Geometry: see drawing. Coordinates: mm, zero at the bounding-box minimum. Round coordinates to 2 decimals unless told otherwise and drop trailing zeros. Loops run counter-clockwise (first coordinate to the right, second up) from the corner with the lowest first, then second, coordinate; pieces in that order, holes last. Notation, with made-up numbers: (61.5, 43) - (77.5, 43) arc R15 cw to (77.5, 67) - close; hole circle Ø5 at (-19, -35). An arc over 180 degrees is marked (long way). Return JSON: item names as keys, results as strings. Group by question number.
1. Section B-B on y = 1. Return loops of the section in (x, z), and give its area (3 significant figures).
2. Section A-A on y = 6.25. Return loops of the section in (x, z).
3. First-contact query: pin 1 Ø1 at (y, z) = (3, 12.5) entering from -X; pin 2 Ø1 at (y, z) = (2.5, 3.5) entering from -X. Flat tips, straight axial feed; report the tip coordinate or a pass-through.
4. Draft query along Z for the marked faces 1, 2, 3 and 4. Return one class per face: +Z half, -Z half, draft (parallel to the pull), parting line (faces both ways), or undercut.
5. Material intervals for probe 1 along Z at (x, y) = (7.5, 4.6); probe 2 along Y at (x, z) = (8.5, 7); probe 3 along X at (y, z) = (5.5, 9.5), sorted ascending.
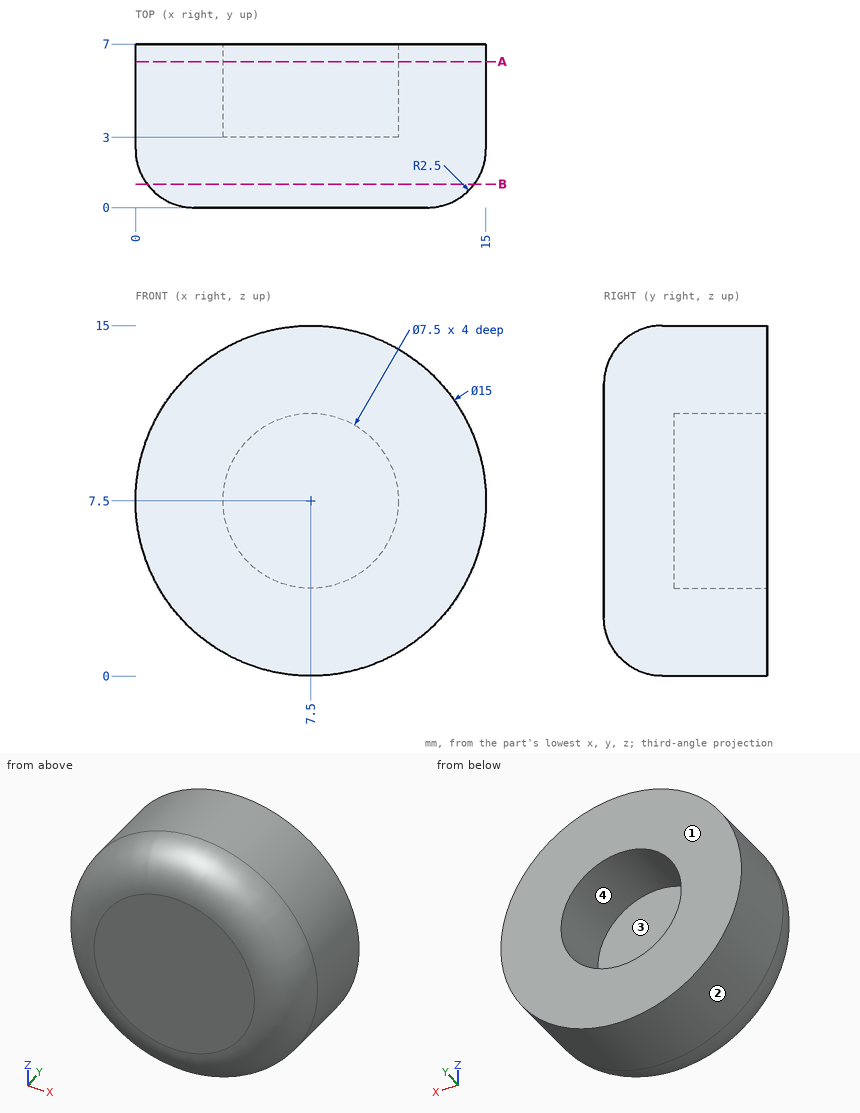
Taken from the geometry:
{
 "1": {"outline": "circle Ø14 at (7.5, 7.5)", "area": "154 mm2"},
 "2": {"outline": "circle Ø15 at (7.5, 7.5); hole circle Ø7.5 at (7.5, 7.5)"},
 "3": {"pin 1": "x = 1.5", "pin 2": "x = 0.87"},
 "4": {"face 1": "draft", "face 2": "parting line", "face 3": "undercut", "face 4": "undercut"},
 "5": {"probe 1": "0 to 3.75, 11.25 to 15", "probe 2": "0 to 3", "probe 3": "0.27 to 4.33, 10.67 to 14.73"}
}
